Geometry check sheet. Reference: the model listing, model coordinates, mm. A direction names the side the tool comes from. Coordinates: 2 decimals unless noted, no trailing zeros. Order: outer loops, then holes, each group sorted by start corner. A loop starts at its lowest first (then second) coordinate and runs counter-clockwise, first axis right, second up. Notation, with made-up numbers: M -31,45.25 L 28,45.25 A31 cw 28,74.25 Z; hole C 55,11 d6. An arc over 180 degrees is marked long. One line per item, written item: value. Start each with the question number.
1) Sectioned sample at C-C, the plane x = -42. Enter the section's corners in (y, z), then the cut area to 3 significant figures.
2) Go/stop test with flat-tipped pins: P1, Ø3.5, axis at y = 46.5, z = 20, coming from the -X side; P2, Ø2, axis at x = -28.5, z = 27.5, coming from the -Y side; P3, Ø8, axis at x = 7.5, y = 39, coming from the +Z side; P4, Ø1, axis at x = 2.5, z = -34, coming from the +Y side. Record where each tip stops, or that it passes through.
3) Draft check along Z on faces 4 (the flat face through (-27, 2, 33)), 5 (the cylindrical face through (-1.496, 30.737, -40.14)), 6 (the flat face through (22, 29, -30)), 7 (the flat face through (-6, 35, 21)). Enter one of: pulls with the +Z half, pulls with the -Z half, needs draft (parallel to the pull), parting line crosses it, or undercut.
4) Thickness scan on L1, parallel to Z at x = -8, y = 27; L2, parallel to X at y = 44.5, z = 20; L3, parallel to Y at x = -57.5, z = 27.25. Record the ranges inside material, lowest first. Write a range as from..to.
5) Sectioned sample at B-B, the plane z = -18. Enter the section's corners in (x, y).
6) Access from +Z, -Z, +X, -X, +Y, -Y to the whole of each face (thin tool, end or side, straight path). Record for faces 1 (the cylindrical face through (-48, 35, 24)), 2 (the flat face through (15, 37, 9.85)), 3 (the flat face through (28, 36, 34)).
7) Sectioned sample at A-A, the plane x = -57.5. Enter the section's corners in (y, z).
```python
from build123d import *

# Parameters (mm, degrees)
SKETCH5_W            = 30
SKETCH5_H            = 30
BOSS_EXTRUDE3_DEPTH  = 72
CUT_EXTRUDE1_DEPTH   = 84.570329663
SKETCH8_W            = 4.95
SKETCH8_H            = 6
CUT_EXTRUDE3_DEPTH   = 84.570329663
SKETCH10_W           = 3
SKETCH10_H           = 72
BOSS_EXTRUDE4_DEPTH  = 10
SKETCH11_W           = 37
SKETCH11_H           = 37
BOSS_EXTRUDE5_DEPTH  = 50
SKETCH14_R           = 1.5
CUT_EXTRUDE4_DEPTH   = 20
FILLET2_R            = 15
SKETCH16_W           = 5
SKETCH16_H           = 72
BOSS_EXTRUDE6_DEPTH  = 73
BOSS_EXTRUDE7_DEPTH  = 8
SKETCH20_W           = 103
SKETCH20_H           = 2
BOSS_EXTRUDE8_DEPTH  = 1.5
SKETCH21_W           = 103
SKETCH21_H           = 2
BOSS_EXTRUDE9_DEPTH  = 1.5
SKETCH22_W           = 15
SKETCH22_H           = 7
BOSS_EXTRUDE10_DEPTH = 72
FILLET4_R            = 5
FILLET5_R            = 3
FILLET6_R            = 2
SKETCH23_R           = 1.5
CUT_EXTRUDE5_DEPTH   = 124.032516027
SKETCH24_W           = 3
SKETCH24_H           = 72
BOSS_EXTRUDE11_DEPTH = 10


with BuildPart() as part:
    # Sketch5 → Boss-Extrude3 (new body)
    with BuildSketch(Plane(origin=(0, 0, 0), x_dir=(1, 0, 0), z_dir=(0, 1, 0))):
        with Locations((15, -15)):
            Rectangle(SKETCH5_W, SKETCH5_H)
    extrude(amount=BOSS_EXTRUDE3_DEPTH)

    # Sketch6 → Cut-Extrude1 (cut, through all)
    with BuildSketch(Plane(origin=(0, 72, 0), x_dir=(1, 0, 0), z_dir=(0, 1, 0))):
        Polygon((12.25, -4.95), (4.95, -4.95), (4.95, -15), (20.15, -15), (20.15, -12.25), (23.05, -10.25), (23.05, -12.25), (25.05, -12.25), (25.05, -4.95), (17.75, -4.95), (17.75, -6.95), (19.75, -6.95), (17.75, -9.85), (12.25, -9.85), (10.25, -6.95), (12.25, -6.95), align=None)
        Polygon((20.15, -15), (4.95, -15), (4.95, -25.05), (12.25, -25.05), (12.25, -23.05), (10.25, -23.05), (12.25, -20.15), (17.75, -20.15), (19.75, -23.05), (17.75, -23.05), (17.75, -25.05), (25.05, -25.05), (25.05, -17.75), (23.05, -17.75), (23.05, -19.75), (20.15, -17.75), align=None)
    extrude(amount=-CUT_EXTRUDE1_DEPTH, mode=Mode.SUBTRACT)

    # Sketch8 → Cut-Extrude3 (cut, through all)
    with BuildSketch(Plane(origin=(0, 72, 0), x_dir=(1, 0, 0), z_dir=(0, 1, 0))):
        with Locations((2.475, -15)):
            Rectangle(SKETCH8_W, SKETCH8_H)
    extrude(amount=-CUT_EXTRUDE3_DEPTH, mode=Mode.SUBTRACT)

    # Sketch10 → Boss-Extrude4 (add)
    with BuildSketch(Plane.ZY):
        with Locations((1.5, 36)):
            Rectangle(SKETCH10_W, SKETCH10_H)
        with Locations((10.5, 36)):
            Rectangle(SKETCH10_W, SKETCH10_H)
        with Locations((19.5, 36)):
            Rectangle(SKETCH10_W, SKETCH10_H)
    extrude(amount=BOSS_EXTRUDE4_DEPTH)

    # Sketch11 → Boss-Extrude5 (add)
    with BuildSketch(Plane(origin=(0, 0, 0), x_dir=(-1, 0, 0), z_dir=(0, 0, -1))):
        with Locations((-10, 36)):
            Rectangle(SKETCH11_W, SKETCH11_H)
    extrude(amount=BOSS_EXTRUDE5_DEPTH)

    # Sketch14 → Cut-Extrude4 (cut)
    with BuildSketch(Plane(origin=(0, 0, -50), x_dir=(-1, 0, 0), z_dir=(0, 0, -1))):
        with Locations((-10, 49.5)):
            Circle(SKETCH14_R)
        with Locations((1.691342951, 29.25)):
            Circle(SKETCH14_R)
        with Locations((-21.691342951, 29.25)):
            Circle(SKETCH14_R)
    extrude(amount=-CUT_EXTRUDE4_DEPTH, mode=Mode.SUBTRACT)

    # Fillet2
    fillet2_edges = [part.edges().sort_by_distance(p)[0] for p in [
        (28.5, 54.5, -25),
        (28.5, 17.5, -25),
        (-8.5, 17.5, -25),
        (-8.5, 54.5, -25),
    ]]
    fillet(fillet2_edges, radius=FILLET2_R)

    # Sketch16 → Boss-Extrude6 (add)
    with BuildSketch(Plane.ZY):
        with Locations((27.5, 36)):
            Rectangle(SKETCH16_W, SKETCH16_H)
    extrude(amount=BOSS_EXTRUDE6_DEPTH)

    # Sketch19 → Boss-Extrude7 (add)
    with BuildSketch(Plane.XY.offset(30)):
        Polygon((-73, 72), (-73, 70), (17.393398282, 70), (28, 59.393398282), (28, 12.606601718), (17.393398282, 2), (-73, 2), (-73, 0), (30, 0), (30, 72), align=None)
    extrude(amount=BOSS_EXTRUDE7_DEPTH)

    # Sketch20 → Boss-Extrude8 (add)
    with BuildSketch(Plane.XZ.offset(-70)):
        with Locations((-21.5, 37)):
            Rectangle(SKETCH20_W, SKETCH20_H)
    extrude(amount=BOSS_EXTRUDE8_DEPTH)

    # Sketch21 → Boss-Extrude9 (add)
    with BuildSketch(Plane(origin=(0, 2, 0), x_dir=(1, 0, 0), z_dir=(0, 1, 0))):
        with Locations((-21.5, -37)):
            Rectangle(SKETCH21_W, SKETCH21_H)
    extrude(amount=BOSS_EXTRUDE9_DEPTH)

    # Sketch22 → Boss-Extrude10 (add)
    with BuildSketch(Plane(origin=(0, 72, 0), x_dir=(1, 0, 0), z_dir=(0, 1, 0))):
        with Locations((-57.5, -21.5)):
            Rectangle(SKETCH22_W, SKETCH22_H)
    extrude(amount=-BOSS_EXTRUDE10_DEPTH)

    # Fillet4
    fillet4_edges = [part.edges().sort_by_distance(p)[0] for p in [
        (-65, 36, 25),
        (-50, 36, 25),
    ]]
    fillet(fillet4_edges, radius=FILLET4_R)

    # Fillet5
    fillet5_edges = [part.edges().sort_by_distance(p)[0] for p in [
        (0, 36, 3),
        (0, 36, 9),
    ]]
    fillet(fillet5_edges, radius=FILLET5_R - 0.0001)  # a hair under: the kernel refuses the full size

    # Fillet6
    fillet6_edges = [part.edges().sort_by_distance(p)[0] for p in [
        (0, 36, 21),
        (0, 36, 25),
    ]]
    fillet(fillet6_edges, radius=FILLET6_R - 0.0001)  # a hair under: the kernel refuses the full size

    # Sketch23 → Cut-Extrude5 (cut, through all)
    with BuildSketch(Plane(origin=(0, 0, 18), x_dir=(-1, 0, 0), z_dir=(0, 0, -1))):
        with Locations((57.5, 61)):
            Circle(SKETCH23_R)
        with Locations((57.5, 11)):
            Circle(SKETCH23_R)
    extrude(amount=-CUT_EXTRUDE5_DEPTH, mode=Mode.SUBTRACT)

    # Sketch24 → Boss-Extrude11 (add)
    with BuildSketch(Plane.ZY.offset(10)):
        with Locations((1.5, 36)):
            Rectangle(SKETCH24_W, SKETCH24_H)
        with Locations((10.5, 36)):
            Rectangle(SKETCH24_W, SKETCH24_H)
    extrude(amount=BOSS_EXTRUDE11_DEPTH)


solid = part.part
```
Final values:
1. outline: M 0,25 L 72,25 L 72,38 L 68.5,38 L 68.5,36 L 70,36 L 70,30 L 2,30 L 2,36 L 3.5,36 L 3.5,38 L 0,38 Z
1. area: 398 mm^2
2. P1: stops at x = -65.32
2. P2: stops at y = 0
2. P3: stops at z = 30
2. P4: stops at y = 54.09
3. face 4: undercut
3. face 5: needs draft
3. face 6: pulls with the -Z half
3. face 7: undercut
4. L1: z = 0..3, 9..12, 18..21, 25..30
4. L2: x = -65..-50, -10..4.95, 25.05..30
4. L3: y = 0..9.5, 12.5..59.5, 62.5..72
5. outline: M -8.5,32.5 A15 ccw 6.5,17.5 L 13.5,17.5 A15 ccw 28.5,32.5 L 28.5,39.5 A15 ccw 13.5,54.5 L 6.5,54.5 A15 ccw -8.5,39.5 Z
6. face 1: -Z, +Y, -Y
6. face 2: +Y, -Y
6. face 3: +Z, -X
7. outline: M 0,18 L 9.5,18 L 9.5,30 L 2,30 L 2,36 L 3.5,36 L 3.5,38 L 0,38 Z; M 12.5,18 L 59.5,18 L 59.5,30 L 12.5,30 Z; M 62.5,18 L 72,18 L 72,38 L 68.5,38 L 68.5,36 L 70,36 L 70,30 L 62.5,30 Z
